```python
from build123d import *
from build123d.topology import SkipClean

# Parameters (mm, degrees)
BOSS_EXTRUDE1_START = 10
SKETCH1_R           = 45
BOSS_EXTRUDE1_DEPTH = 5
BOSS_EXTRUDE3_DEPTH = 10
CIRPATTERN1_COUNT   = 2
CIRPATTERN1_ANGLE   = 90
SKETCH5_OUTSIDE_W   = 124.038
SKETCH5_OUTSIDE_H   = 124.038
SKETCH5_OUTSIDE_R   = 45
CUT_EXTRUDE1_DEPTH  = 69.82949949
CHAMFER1_START      = -45
CHAMFER1_2_DEPTH    = 42.5
CHAMFER1_START_2    = 2.5
CHAMFER1_3_DEPTH    = 42.5
CHAMFER1_4_DEPTH    = 42.5
CHAMFER1_5_DEPTH    = 42.5
FILLET1_R           = 5
SKETCH6_R           = 5
CUT_EXTRUDE2_DEPTH  = 65.420493634
CIRPATTERN2_COUNT   = 4


with BuildPart() as part:
    # Sketch1 → Boss-Extrude1 (new body)
    with BuildSketch(Plane(origin=(0, 0, 0), x_dir=(0, 1, 0), z_dir=(0, 0, 1)).offset(BOSS_EXTRUDE1_START)):
        with Locations(Location((0, 0, 0), (0, 0, 270))):
            Circle(SKETCH1_R)
    extrude(amount=BOSS_EXTRUDE1_DEPTH)

    # Sketch4 → Boss-Extrude3 (add)
    with BuildSketch(Plane.XY.offset(15)):
        with BuildLine():
            Line((-2.5, -45), (-2.5, 45))
            ThreePointArc((-2.5, 45), (0, 47.5), (2.5, 45))
            Line((2.5, 45), (2.5, -45))
            ThreePointArc((2.5, -45), (0, -47.5), (-2.5, -45))
        make_face()
    boss_extrude3 = extrude(amount=BOSS_EXTRUDE3_DEPTH)

    # CirPattern1: Boss-Extrude3 ×2 about axis
    cirpattern1_axis = Axis((0, 0, 0), (0, 0, 1))
    for i in range(1, CIRPATTERN1_COUNT):
        add(boss_extrude3.rotate(cirpattern1_axis, i * CIRPATTERN1_ANGLE / (CIRPATTERN1_COUNT - 1)))

    # Sketch5 outside → Cut-Extrude1 (cut, through all)
    with SkipClean():  # the faces are left unmerged after this step: merging them gives an invalid solid
        with BuildSketch(Plane(origin=(0, 0, 10), x_dir=(1, 0, 0), z_dir=(0, 0, -1))):
            Rectangle(SKETCH5_OUTSIDE_W, SKETCH5_OUTSIDE_H)
            with Locations(Location((0, 0, 0), (0, 0, 183.184738537))):
                Circle(SKETCH5_OUTSIDE_R, mode=Mode.SUBTRACT)
        extrude(amount=-CUT_EXTRUDE1_DEPTH, mode=Mode.SUBTRACT)

    # Chamfer1: read off the stored shape, not the designer's step
    # Chamfer1 outline → Chamfer1 (revolve, cut)
    with BuildSketch(Plane.XZ):
        Polygon((45, 25), (41.360297657, 25), (45, 15), align=None)
    revolve(axis=Axis((0, 0, 0), (0, 0, 1)), mode=Mode.SUBTRACT)

    # Chamfer1 2 outline → Chamfer1 2 (cut)
    with BuildSketch(Plane(origin=(0, 0, 0), x_dir=(1, 0, 0), z_dir=(0, 1, 0)).offset(CHAMFER1_START)):
        Polygon((2.5, -15), (-1.139702343, -25), (2.5, -25), align=None)
    extrude(amount=CHAMFER1_2_DEPTH, mode=Mode.SUBTRACT)

    # Chamfer1 3 outline → Chamfer1 3 (cut)
    with BuildSketch(Plane(origin=(0, 0, 0), x_dir=(1, 0, 0), z_dir=(0, 1, 0)).offset(CHAMFER1_START_2)):
        Polygon((-2.5, -15), (-2.5, -25), (1.139702343, -25), align=None)
    extrude(amount=CHAMFER1_3_DEPTH, mode=Mode.SUBTRACT)

    # Chamfer1 4 outline → Chamfer1 4 (cut)
    with BuildSketch(Plane.YZ.offset(CHAMFER1_START)):
        Polygon((-2.5, 15), (1.139702343, 25), (-2.5, 25), align=None)
    extrude(amount=CHAMFER1_4_DEPTH, mode=Mode.SUBTRACT)

    # Chamfer1 5 outline → Chamfer1 5 (cut)
    with BuildSketch(Plane.YZ.offset(CHAMFER1_START_2)):
        Polygon((2.5, 15), (2.5, 25), (-1.139702343, 25), align=None)
    extrude(amount=CHAMFER1_5_DEPTH, mode=Mode.SUBTRACT)

    # Fillet1
    fillet1_edges = [part.edges().sort_by_distance(p)[0] for p in [
        (-0.680148828, 2.5, 20),
        (2.5, 0.680148828, 20),
        (0.680148829, -2.5, 20),
        (-2.5, -0.680148829, 20),
    ]]
    fillet(fillet1_edges, radius=FILLET1_R)

    # Sketch6 → Cut-Extrude2 (cut, through all)
    with BuildSketch(Plane.XY.offset(15)):
        with Locations((-30.310889132, 17.5)):
            Circle(SKETCH6_R)
        with Locations((-17.5, 30.310889132)):
            Circle(SKETCH6_R)
        with Locations((-12.810889132, 12.810889132)):
            Circle(SKETCH6_R)
    cut_extrude2 = extrude(amount=-CUT_EXTRUDE2_DEPTH, mode=Mode.SUBTRACT)

    # CirPattern2: Cut-Extrude2 ×4 about axis
    cirpattern2_axis = Axis((0, 0, 0), (0, 0, 1))
    for i in range(1, CIRPATTERN2_COUNT):
        add(cut_extrude2.rotate(cirpattern2_axis, i * 360 / CIRPATTERN2_COUNT), mode=Mode.SUBTRACT)


solid = part.part
```
Geometry: final body of the model. Coordinates: model frame, mm. A direction names the side the tool comes from. Coordinates: 2 decimals unless noted, no trailing zeros. Order: outer loops, then holes, each group sorted by start corner. A loop starts at its lowest first (then second) coordinate and runs counter-clockwise, first axis right, second up.
Item 1: Section query A-A (x = 19). Output: boundary loops of the cut face in (y, z).
Answer:
outline: (-40.79, 10) - (-35.08, 10) - (-35.08, 15) - (-40.79, 15) - close; (-25.54, 10) - (25.54, 10) - (25.54, 15) - (2.5, 15) - (-1.14, 25) - (-2.5, 25) - (-2.5, 15) - (-25.54, 15) - close; (35.08, 10) - (40.79, 10) - (40.79, 15) - (35.08, 15) - close
Item 2: Contact query for flat-ended pins moving along their axis: P1, Ø11.5, axis at x = -30.31, y = 17.5, coming from the +Z side; P2, Ø3, axis at y = 30, z = 14.5, coming from the +X side; P3, Ø3, axis at y = -34.5, z = 22, coming from the +X side; P4, Ø8, axis at x = 12.81, y = 12.81, coming from the +Z side. Output: stop coordinate, or through.
Answer:
P1: stops at z = 15
P2: stops at x = 34.82
P3: stops at x = 0.5
P4: passes through
Item 3: Material intervals for line 1 along Y through (x, z) = (-16, 14.5); line 2 along Y through (x, z) = (21, 13.75); line 3 along Z through (x, y) = (-21.5, -6.5), sorted ascending.
Answer:
line 1: y = -42.06 to -35.08, -25.54 to -16.66, -8.96 to 8.96, 16.66 to 25.54, 35.08 to 42.06
line 2: y = -39.8 to -33.88, -26.74 to 26.74, 33.88 to 39.8
line 3: z = 10 to 15
Item 4: Draft query along X for faces 6 (the face through (19, -19, 15)), 7 (the face through (-2.43, 3.93, 19.58)), 8 (the face through (25.692, -15.585, 12.535)), 9 (the face through (-18.15, 35.27, 12.54)). Return one class per face: released by +X, released by -X, zero draft, split by the parting line, or undercut.
Answer:
face 6: zero draft
face 7: released by -X
face 8: undercut
face 9: undercut
Item 5: Section query C-C (z = 12.75). State how many separate pieces and enclosed holes the cut face has, then the cut area to 3 significant figures.
Answer:
separate pieces: 1
enclosed holes: 12
area: 5,420 mm2
Item 6: Access query for faces 1 (the face through (0.705, 43.604, 18.819)), 2 (the face through (19, 19, 15)), 3 (the face through (-0.655, 25.953, 20.07)), 4 (the face through (-2.5, -25, 20)), 5 (the face through (-25.692, 15.585, 12.535)). Directions: +Z, -Z, +X, -X, +Y, -Y. A direction counts if a zero-diameter tool reaches every point of the face in a straight line with its end or side. Return the directions, or none.
Answer:
face 1: +Z, +Y
face 2: +Z, +X, +Y
face 3: +Z, -X, +Y
face 4: +Z, -X, -Y
face 5: +Z, -Z
Item 7: Section query D-D (x = -37). Output: boundary loops of the cut face in (y, z).
Answer:
outline: (-25.61, 10) - (25.61, 10) - (25.61, 15) - (2.5, 15) - (2.5, 25) - (1.14, 25) - (-2.5, 15) - (-25.61, 15) - close
Item 8: Section query B-B (y = -20). Output: boundary loops of the cut face in (x, z), then the cut area to 3 significant figures.
Answer:
outline: (-40.31, 10) - (-34.64, 10) - (-34.64, 15) - (-40.31, 15) - close; (-25.98, 10) - (25.98, 10) - (25.98, 15) - (2.5, 15) - (-1.14, 25) - (-2.5, 25) - (-2.5, 15) - (-25.98, 15) - close; (34.64, 10) - (40.31, 10) - (40.31, 15) - (34.64, 15) - close
area: 348 mm2
